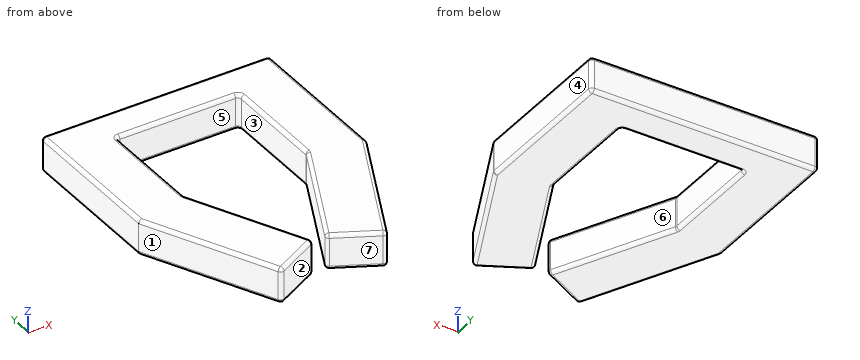
from build123d import *

# Parameters (mm, degrees)
BOSS_EXTRUDE1_DEPTH = 10
FILLET1_R           = 1


with BuildPart() as part:
    # Sketch1 → Boss-Extrude1 (new body)
    with BuildSketch(Plane.XY):
        Polygon((0, 40), (0, 36.611522599), (17.430453908, 0), (30.708058647, 7.006255421), (15, 40), (15, 70), (50, 70), (50, 40), (34.291941353, 7.006255421), (47.569546092, 0), (65, 36.611522599), (65, 80), (0, 80), align=None)
    extrude(amount=BOSS_EXTRUDE1_DEPTH)

    # Fillet1
    fillet1_edges = [part.edges().sort_by_distance(p)[0] for p in [
        (15, 55, 10),
        (24.069256278, 3.50312771, 0),
        (8.715226954, 18.3057613, 0),
        (0, 58.3057613, 0),
        (32.5, 80, 0),
        (65, 58.3057613, 0),
        (32.5, 70, 10),
        (56.284773046, 18.3057613, 0),
        (40.930743722, 3.50312771, 0),
        (42.145970676, 23.50312771, 0),
        (50, 55, 0),
        (32.5, 70, 0),
        (15, 55, 0),
        (22.854029324, 23.50312771, 0),
        (50, 55, 10),
        (30.708058647, 7.006255421, 5),
        (17.430453908, 0, 5),
        (0, 80, 5),
        (65, 80, 5),
        (65, 36.611522599, 5),
        (47.569546092, 0, 5),
        (34.291941353, 7.006255421, 5),
        (50, 40, 5),
        (50, 70, 5),
        (15, 70, 5),
        (15, 40, 5),
        (42.145970676, 23.50312771, 10),
        (40.930743722, 3.50312771, 10),
        (56.284773046, 18.3057613, 10),
        (65, 58.3057613, 10),
        (32.5, 80, 10),
        (0, 58.3057613, 10),
        (8.715226954, 18.3057613, 10),
        (22.854029324, 23.50312771, 10),
        (24.069256278, 3.50312771, 10),
    ]]
    fillet(fillet1_edges, radius=FILLET1_R)


solid = part.part
The listing builds one solid part. Answer for the finished solid, in the listing's coordinates (mm). Face numbers are marked on the shaded views. A direction names the side the tool comes from. Round coordinates to 2 decimals unless told otherwise and drop trailing zeros. Write each loop counter-clockwise with the first axis right and the second up, starting at its lowest first coordinate (ties: lowest second). Pieces come first, ordered by that corner, then holes. Notation, with made-up numbers: (11, -4) - (20, -4) arc R22 ccw to (20, 29) - close; hole circle Ø2 at (82, -9.5). An arc over 180 degrees is marked (long way). Use one line per item in the form item = value. Start each with the question number.
Item 1: A cutting plane is placed at A-A (y = 60). Write down the section's boundary in (x, z), plus the area to 3 significant figures.
Item 2: A cutting plane is placed at B-B (z = 5). Write down the section's boundary in (x, y), plus the area to 3 significant figures.
Item 3: Flat-ended cylindrical pins translate along their axes: pin 1 Ø6 at (x, y) = (27.5, 25.5) entering from +Z; pin 2 Ø1.5 at (x, z) = (51, 4.5) entering from -Y; pin 3 Ø1 at (y, z) = (28, 3.5) entering from -X; pin 4 Ø1.5 at (x, y) = (49.5, 59) entering from +Z. Find the tip coordinate at first contact, or state that the pin passes through.
Item 4: A tool of negligible diameter and unlimited length cuts with its end or side. For the marked faces 1, 2 and 3, from which of +Z, -Z, +X, -X, +Y, -Y can it reach the whole face along a straight path? Write none if from no direction.
Item 5: Determine the mould class of the marked faces 4, 5, 6 and 7 for opening direction Y: +Y half, -Y half, draft (parallel to the pull), parting line (faces both ways), or undercut.
Item 6: Find the intervals of material crossed by line 1 (X direction, y = 41, z = 6); line 2 (Y direction, x = 42, z = 1.75); line 3 (X direction, y = 39.5, z = 2), in increasing order. Write a range as [from, to].
The answers:
q1.outline = (0, 1) arc R1 ccw to (1, 0) - (14, 0) arc R1 ccw to (15, 1) - (15, 9) arc R1 ccw to (14, 10) - (1, 10) arc R1 ccw to (0, 9) - close; (50, 1) arc R1 ccw to (51, 0) - (64, 0) arc R1 ccw to (65, 1) - (65, 9) arc R1 ccw to (64, 10) - (51, 10) arc R1 ccw to (50, 9) - close
q1.area = 298 mm^2
q2.outline = (0, 36.61) - (16.98, 0.94) arc R1 ccw to (18.35, 0.49) - (29.86, 6.56) arc R1 ccw to (30.3, 7.87) - (15.1, 39.8) arc R1 cw to (15, 40.23) - (15, 69) arc R1 cw to (16, 70) - (49, 70) arc R1 cw to (50, 69) - (50, 40.23) arc R1 cw to (49.9, 39.8) - (34.7, 7.87) arc R1 ccw to (35.14, 6.56) - (46.65, 0.49) arc R1 ccw to (48.02, 0.94) - (64.9, 36.41) arc R1 ccw to (65, 36.84) - (65, 79) arc R1 ccw to (64, 80) - (1, 80) arc R1 ccw to (0, 79) - close
q2.area = 2,760 mm^2
q3.pin_1 = through
q3.pin_2 = 5.63
q3.pin_3 = 3.86
q3.pin_4 = 9.66
q4.face_1 = +Z, -Z, -X, -Y
q4.face_2 = +Z, -Z, -Y
q4.face_3 = +Z, -Z
q5.face_4 = draft
q5.face_5 = undercut
q5.face_6 = undercut
q5.face_7 = -Y half
q6.line_1 = [0, 15], [50, 65]
q6.line_2 = [2.94, 23.2], [70, 80]
q6.line_3 = [0, 15.24], [49.76, 65]
